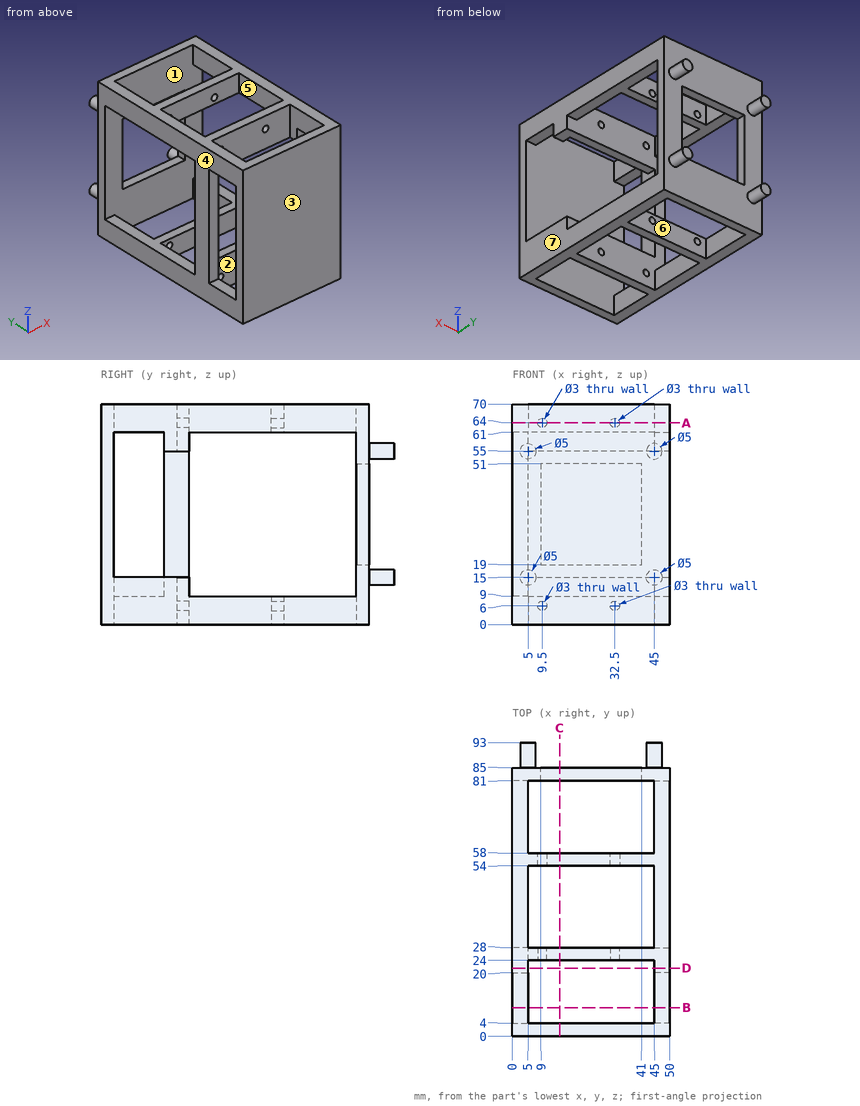
Part print with two shaded views. Sizes in mm from the minimum x, y, z corner. A direction names the side the tool comes from. Round coordinates to 2 decimals unless told otherwise and drop trailing zeros. Write each loop counter-clockwise with the first axis right and the second up, starting at its lowest first coordinate (ties: lowest second). Pieces come first, ordered by that corner, then holes. Notation, with made-up numbers: M 15.5,7 L 44.5,7 A12 cw 44.5,25 Z; hole C 75,4.5 d11. An arc over 180 degrees is marked long. Put each result on its own line as item: value. Start each with the question number.
1) Saw through at C-C, the plane x = 15. Write the cut outline in (y, z), and give its area (3 significant figures).
2) Pull direction X, two halves, no side cores. Call the marked faces 4, 5, 6 and 7: pulls with the +X half, pulls with the -X half, needs draft (parallel to the pull), parting line crosses it, or undercut.
3) Drill centre lines: probe 1 along X at (y, z) = (55.75, 64); probe 2 along Y at (x, z) = (4, 52.5); probe 3 along Y at (x, z) = (19, 63.5). Where is each one in solid material? Low to high. Write a range as [from, to].
4) Pin check, flat tips, straight feed: pin 1 Ø4.5 at (x, z) = (19, 67.5) entering from +Y; pin 2 Ø12 at (y, z) = (54, 15.5) entering from +X. Stop position of each tip, or through.
5) Saw through at A-A, the plane z = 64. Count the separate pieces of the cut face and the enclosed holes in it, and give its area (3 significant figures).
6) Saw through at D-D, the plane y = 21.5. Write the cut outline in (x, z), and give its area (3 significant figures).
7) Saw through at B-B, the plane y = 9. Write the cut outline in (x, z).
8) 3-axis set-ups, long thin cutter, end or side, ignore diameter. For the marked faces 1, 2 and 3: which of +Z, -Z, +X, -X, +Y, -Y reach the whole face in a straight line?
Resolved:
1. outline: M 0,0 L 4,0 L 4,70 L 0,70 Z; M 24,0 L 28,0 L 28,15 L 24,15 Z; M 24,55 L 28,55 L 28,70 L 24,70 Z; M 54,0 L 58,0 L 58,9 L 54,9 Z; M 54,61 L 58,61 L 58,70 L 54,70 Z; M 81,0 L 85,0 L 85,19 L 81,19 Z; M 81,51 L 85,51 L 85,70 L 81,70 Z
1. area: 624 mm²
2. face 4: pulls with the -X half
2. face 5: undercut
2. face 6: undercut
2. face 7: pulls with the +X half
3. probe 1: [0, 8], [11, 31], [34, 50]
3. probe 2: [0, 4], [20, 28], [81, 85]
3. probe 3: [0, 4], [24, 28], [54, 58], [81, 85]
4. pin 1: y = 85
4. pin 2: through
5. separate pieces: 3
5. enclosed holes: 1
5. area: 1,440 mm²
6. outline: M 0,0 L 5,0 L 5,70 L 0,70 Z; M 45,0 L 50,0 L 50,15 L 45,15 Z; M 45,55 L 50,55 L 50,70 L 45,70 Z
6. area: 500 mm²
7. outline: M 0,0 L 5,0 L 5,9 L 0,9 Z; M 0,61 L 5,61 L 5,70 L 0,70 Z; M 45,0 L 50,0 L 50,15 L 45,15 Z; M 45,61 L 50,61 L 50,70 L 45,70 Z
8. face 1: none
8. face 2: +Z, -Z
8. face 3: +Z, -Z, +X, -X, -Y
